```python
from build123d import *

# Parameters (mm, degrees)
CROQUIS1_R              = 7.5
SALIENTE_EXTRUIR2_DEPTH = 50
CROQUIS4_R              = 25
SALIENTE_EXTRUIR3_DEPTH = 3
SALIENTE_EXTRUIR4_START = 25
CROQUIS5_R              = 25
SALIENTE_EXTRUIR4_DEPTH = 3
REDONDEO2_R             = 10


with BuildPart() as part:
    # Croquis1 → Saliente-Extruir2 (new body)
    with BuildSketch(Plane.XY):
        Circle(CROQUIS1_R)
    extrude(amount=SALIENTE_EXTRUIR2_DEPTH)

    # Croquis4 → Saliente-Extruir3 (add)
    with BuildSketch(Plane.XY):
        Circle(CROQUIS4_R)
    extrude(amount=SALIENTE_EXTRUIR3_DEPTH)

    # Croquis5 → Saliente-Extruir4 (add)
    with BuildSketch(Plane.XY.offset(SALIENTE_EXTRUIR4_START)):
        Circle(CROQUIS5_R)
    extrude(amount=SALIENTE_EXTRUIR4_DEPTH)

    # Redondeo2
    redondeo2_edges = [part.edges().sort_by_distance(p)[0] for p in [
        (-7.5, 0, 25),
        (-7.5, 0, 3),
    ]]
    fillet(redondeo2_edges, radius=REDONDEO2_R)


solid = part.part
```
Could you check a few things on this model? Use its own coordinates, in mm. A direction names the side the tool comes from. Round coordinates to 2 decimals unless told otherwise and drop trailing zeros. Loops run counter-clockwise (first coordinate to the right, second up) from the corner with the lowest first, then second, coordinate; pieces in that order, holes last.
Q1. I want a section at B-B (y = 0). Write out the boundary of the cut face in (x, z), and give its area (3 significant figures).
Q2. Thinking about a two-plate mould opening in Z: for faces 1 (the flat face through (-17, -5, 25)), 2 (the flat face through (0, 0, 0)), 3 (the cylindrical face through (-7.493, 0.33, 38.846)), 4 (the flat face through (-6, -5, 28)), which applies, pulls with the +Z half, pulls with the -Z half, needs draft (parallel to the pull), parting line crosses it, or undercut?
Q3. I want a section at A-A (x = -20). Write out the boundary of the cut face in (y, z), and give its area (3 significant figures).
Q4. I want a section at D-D (z = 41). Write out the boundary of the cut face in (x, y), and give its area (3 significant figures).
Q5. For P1, Ø1.5, axis at y = -6, z = 36.5, coming from the +X side; P2, Ø10, axis at y = 10.5, z = 25.5, coming from the +X side; P3, Ø4, axis at x = -9.5, y = 13.5, coming from the +Z side, each with a flat end and sliding along its axis, tell me the tip position at first contact or that it passes through.
Q6. On a 3-axis mill with a long thin cutter (end or side, diameter ignored), from which of +Z, -Z, +X, -X, +Y, -Y can I reach the whole of each face in a straight line? I mean faces 5 (the cylindrical face through (23.846, 7.509, 1.479)), 6 (the cylindrical face through (-7.493, 0.33, 13.986)). Say none if no direction works.
Q7. Please list where these lines run through material, in increasing order: L1, parallel to Z at x = -0.5, y = 18; L2, parallel to Z at x = 15, y = 6.5; L3, parallel to X at y = 6.5, z = 32.5.
Answer below:
1. outline: (-25, 0) - (25, 0) - (25, 3) - (17.5, 3) arc R10 cw to (7.5, 13) - (7.5, 15) arc R10 cw to (17.5, 25) - (25, 25) - (25, 28) - (7.5, 28) - (7.5, 50) - (-7.5, 50) - (-7.5, 28) - (-25, 28) - (-25, 25) - (-17.5, 25) arc R10 cw to (-7.5, 15) - (-7.5, 13) arc R10 cw to (-17.5, 3) - (-25, 3) - close
1. area: 1,050 mm2
2. face 1: undercut
2. face 2: pulls with the -Z half
2. face 3: needs draft
2. face 4: pulls with the +Z half
3. outline: (-15, 0) - (15, 0) - (15, 3) - (-15, 3) - close; (-15, 25) - (15, 25) - (15, 28) - (-15, 28) - close
3. area: 180 mm2
4. outline: circle Ø15 at (0, 0)
4. area: 177 mm2
5. P1: stops at x = 5.36
5. P2: stops at x = 24.39
5. P3: stops at z = 28
6. face 5: +Z, -Z
6. face 6: none
7. L1: z = 0 to 3, 25 to 28
7. L2: z = 0 to 3.07, 24.93 to 28
7. L3: x = -3.74 to 3.74
